Work out the finished part from the listing and answer in its coordinate system (mm). Face numbers are marked on the shaded views. A direction names the side the tool comes from. Coordinates: 2 decimals unless noted, no trailing zeros. Loops run counter-clockwise (first coordinate to the right, second up) from the corner with the lowest first, then second, coordinate; pieces in that order, holes last.
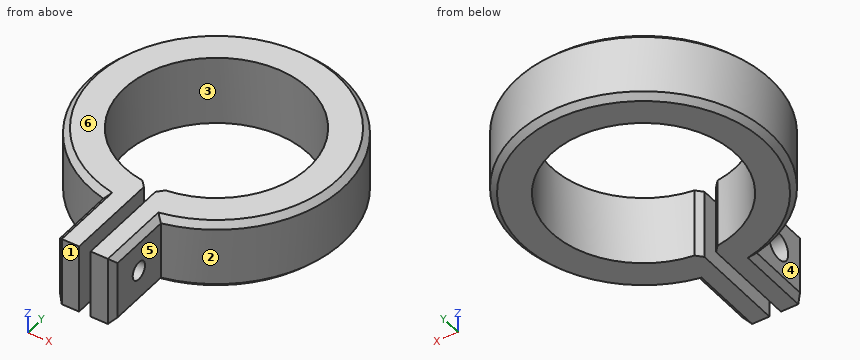
Autodesk Inventor part; units mm, degrees
ref_plane "YZ Plane" through (0, 0, 0) normal (1, 0, 0) x (0, 1, 0)
ref_plane "XZ Plane" through (0, 0, 0) normal (0, 1, 0) x (-1, 0, 0)
ref_plane "XY Plane" through (0, 0, 0) normal (0, 0, 1) x (1, 0, 0)
sketch "Esquisse1" plane through (0, 0, 0) normal (0, 0, 1) x (1, 0, 0)
  arc A0 (0.5, -7.9844) -> (-0.5, -7.9844) centre (0, 0) ccw
  arc A1 (2.5, -10.7121) -> (-2.5, -10.7121) centre (0, 0) ccw
  line L0 (-0.5, -7.9844) -> (-0.5, -16.7121)
  line L1 (0.5, -7.9844) -> (0.5, -16.7121)
  line L2 (-0.5, -7.9844) -> (0.5, -7.9844) construction
  line L3 (-0.5, -16.7121) -> (-2.5, -16.7121)
  line L4 (-2.5, -16.7121) -> (-2.5, -10.7121)
  line L5 (0.5, -16.7121) -> (2.5, -16.7121)
  line L6 (2.5, -16.7121) -> (2.5, -10.7121)
  point P0 (0, -7.9844)
  dimension "d0" = 8
  dimension "d1" = 1
  dimension "d2" = 3
  dimension "d3" = 6
  dimension "d4" = 2
extrude "Extrusion1" add sketch "Esquisse1" along normal blind 6
chamfer "Chanfrein1" distance 0.5 angle 45 10 edges at (0, 11, 6) (0, 11, 0) (-2.5, -16.7121, 3) (2.5, -16.7121, 3) (2.5, -13.7121, 6) (2.5, -13.7121, 0) (-2.5, -13.7121, 6) (-2.5, -13.7121, 0) (-0.5, -7.9844, 3) (0.5, -7.9844, 3)
sketch "Esquisse2" plane through (-2.5, -16.2121, 0.5) normal (-1, 0, 0) x (0, 0, 1)
  line L0 (-0.5, -0.5) -> (5.5, -0.5)
  line L1 (5.5, -0.5) -> (5.5, 5.9044)
  point P0 (-0.5, 16.2121)
  point P1 (2.5, 2.7022)
  point P2 (2.5, -0.5)
  point P3 (5.5, 2.7022)
hole "Perçage1" at (-2.5, -13.51, 3) direction (1, 0, 0) diameter 2.4 depth 2
sketch "Esquisse3" plane through (2.5, -16.2121, 0.5) normal (1, 0, 0) x (0, 0, -1)
  line L0 (0.5, -0.5) -> (0.5, 5.9044)
  line L1 (-5.5, -0.5) -> (0.5, -0.5)
  point P0 (0.5, 16.2121)
  point P1 (-2.5, 2.7022)
  point P2 (0.5, 2.7022)
  point P3 (-2.5, -0.5)
hole "Perçage2" at (2.5, -13.51, 3) direction (-1, 0, 0) diameter 1.567 depth 2
properties part number "blocage_ressort_canon" material "Aluminium 6061"
1. A cutting plane is placed at C-C, the plane y = 0. Give the vertices of the cut face in (x, z), then the cut area to 3 significant figures.
2. Straight lines are drawn through the part: probe 1 along Y at (x, z) = (-2, 3.7); probe 2 along Z at (x, y) = (-1.7, -13.51); probe 3 along X at (y, z) = (-11.75, 0.75). For each, find the intervals that lie inside material, in ascending order.
3. Each of these flat-tipped pins is pushed along its axis until it touches: P1, Ø1, axis at y = 4, z = 4.5, coming from the -X side; P2, Ø2, axis at y = -13.51, z = 3, coming from the +X side; P3, Ø1, axis at y = -7, z = 3, coming from the +X side. Where does it stop, or does it pass through?
4. A cutting plane is placed at A-A, the plane y = -12. Give the vertices of the cut face in (x, z).
5. Determine the mould class of the marked faces 1, 2, 3 and 4 for opening direction Y: released by +Y, released by -Y, zero draft, split by the parting line, or undercut.
6. A cutting plane is placed at B-B, the plane z = 3. Give the vertices of the cut face in (x, y).
7. A cutting plane is placed at D-D, the plane z = 1.1. Give the vertices of the cut face in (x, y).
8. For the marked faces 5 and 6, determine the directions among +Z, -Z, +X, -X, +Y, -Y from which every point of the face is accessible in a straight line to the end or side of a thin tool.
Answers below:
1. outline: (-11, 0.5) - (-10.5, 0) - (-8, 0) - (-8, 6) - (-10.5, 6) - (-11, 5.5) - close; (8, 0) - (10.5, 0) - (11, 0.5) - (11, 5.5) - (10.5, 6) - (8, 6) - close
1. area: 35.5 mm2
2. probe 1: y = -16.71 to -14.48, -12.54 to -7.75, 7.75 to 10.82
2. probe 2: z = 0 to 1.8, 4.2 to 6
2. probe 3: x = -2.5 to -0.5, 0.5 to 2.5
3. P1: stops at x = -10.43
3. P2: stops at x = 2.5
3. P3: stops at x = 8.87
4. outline: (-2.5, 0.5) - (-2, 0) - (-0.5, 0) - (-0.5, 6) - (-2, 6) - (-2.5, 5.5) - close; (0.5, 0) - (2, 0) - (2.5, 0.5) - (2.5, 5.5) - (2, 6) - (0.5, 6) - close
5. face 1: released by -Y
5. face 2: split by the parting line
5. face 3: undercut
5. face 4: zero draft
6. outline: (-2.5, -16.21) - (-2, -16.71) - (-0.5, -16.71) - (-0.5, -14.71) - (-2.5, -14.71) - close; (-2.5, -12.31) - (-0.5, -12.31) - (-0.5, -8.48) - (-1, -7.94) arc R8 cw (long way) to (1, -7.94) - (0.5, -8.48) - (0.5, -12.73) - (2.5, -12.73) - (2.5, -10.71) arc R11 ccw (long way) to (-2.5, -10.71) - close; (0.5, -16.71) - (2, -16.71) - (2.5, -16.21) - (2.5, -14.29) - (0.5, -14.29) - close
7. outline: (-2.5, -16.21) - (-2, -16.71) - (-0.5, -16.71) - (-0.5, -8.48) - (-1, -7.94) arc R8 cw (long way) to (1, -7.94) - (0.5, -8.48) - (0.5, -16.71) - (2, -16.71) - (2.5, -16.21) - (2.5, -10.71) arc R11 ccw (long way) to (-2.5, -10.71) - close
8. face 5: +Z, -Z, +X, -Y
8. face 6: +Z, +X, -X, +Y, -Y
